Verification items for this drawing (mm, ordinates from the low corner). Coordinates: 2 decimals unless noted, no trailing zeros. Write each loop counter-clockwise with the first axis right and the second up, starting at its lowest first coordinate (ties: lowest second). Pieces come first, ordered by that corner, then holes. Notation, with made-up numbers: (86, -5) -> (126, -5) arc R11 ccw to (126, 4) -> close; hole circle Ø1 at (35.25, -35). An arc over 180 degrees is marked (long way). Answer as CSV lines item,"result".
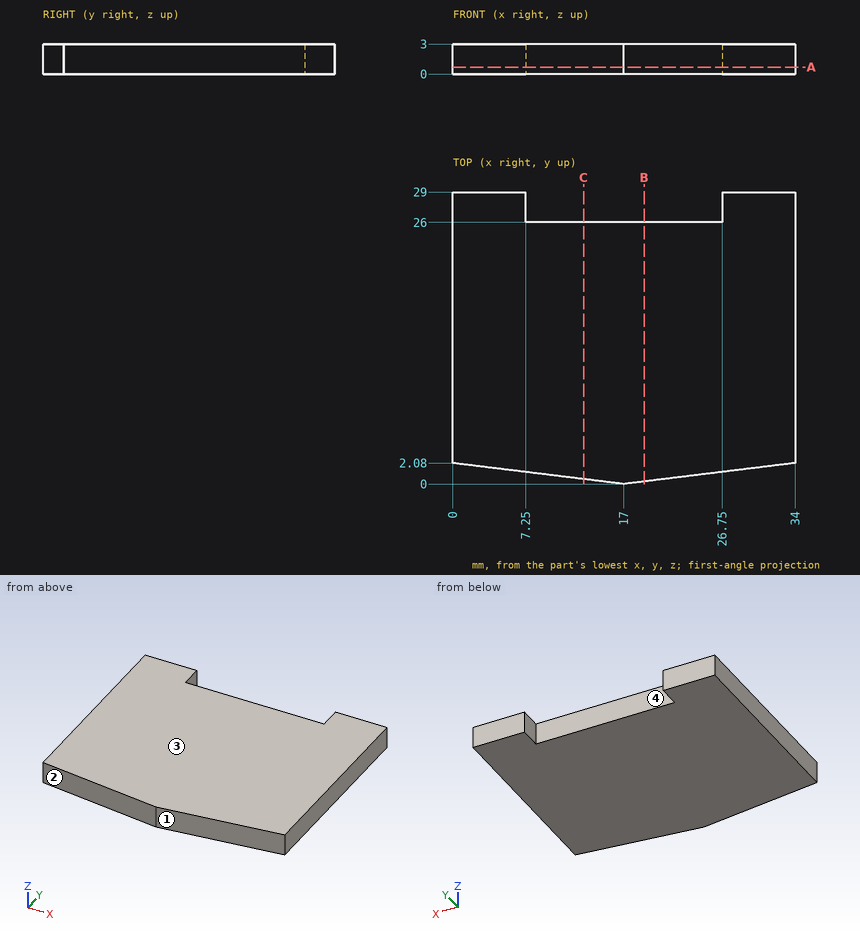
Item 1: Release check for a two-part mould opening along X. For the marked faces 1, 2, 3 and 4 record: +X half, -X half, draft (parallel to the pull), parting line (faces both ways), or undercut.
Responses:
face 1,"+X half"
face 2,"-X half"
face 3,"draft"
face 4,"undercut"
Item 2: Depth check by flat-ended pin: pin 1 Ø1.5 at (x, z) = (18.5, 1.5) entering from +Y; pin 2 Ø1.5 at (x, y) = (20.5, 23.5) entering from -Z. Enter the tip coordinate at first touch or a pass-through.
Responses:
pin 1,"stops at y = 26"
pin 2,"stops at z = 0"
Item 3: Cross-section at A-A, the plane z = 0.7. Record the cut outline in (x, y), plus the area to 3 significant figures.
Responses:
outline,"(0, 2.08) -> (17, 0) -> (34, 2.08) -> (34, 29) -> (26.75, 29) -> (26.75, 26) -> (7.25, 26) -> (7.25, 29) -> (0, 29) -> close"
area,"892 mm2"
Item 4: Cross-section at B-B, the plane x = 19. Record the cut outline in (y, z).
Responses:
outline,"(0.24, 0) -> (26, 0) -> (26, 3) -> (0.24, 3) -> close"
Item 5: Cross-section at C-C, the plane x = 13. Record the cut outline in (y, z), plus the area to 3 significant figures.
Responses:
outline,"(0.49, 0) -> (26, 0) -> (26, 3) -> (0.49, 3) -> close"
area,"76.5 mm2"
Item 6: Thickness scan on probe 1 along X at (y, z) = (27.5, 0.85); probe 2 along Y at (x, z) = (9, 0.4); probe 3 along Y at (x, z) = (21, 1.85). Record the ranges inside material, lowest first.
Responses:
probe 1,"x = 0 to 7.25, 26.75 to 34"
probe 2,"y = 0.98 to 26"
probe 3,"y = 0.49 to 26"
